Verification items for the finished model (mm, model axes). A direction names the side the tool comes from. Round coordinates to 2 decimals unless told otherwise and drop trailing zeros. Loops run counter-clockwise (first coordinate to the right, second up) from the corner with the lowest first, then second, coordinate; pieces in that order, holes last. Notation, with made-up numbers: (80.5, 50) -> (120.5, 50) arc R23 cw to (120.5, 63) -> close; hole circle Ø10 at (12, 26.25). An arc over 180 degrees is marked (long way). Write item = value, one per line. Start each with the question number.
```python
from build123d import *

# Parameters (mm, degrees)
BOSS_EXTRUDE1_DEPTH      = 20
BOSS_EXTRUDE2_DEPTH      = 12.7
BOSS_EXTRUDE2_DEPTH_BACK = 21.59
SKETCH2_R                = 5.710413334
CUT_EXTRUDE1_DEPTH       = 56.401981837


with BuildPart() as part:
    # Sketch1 → Boss-Extrude1 (new body)
    with BuildSketch(Plane(origin=(0, 0, 0), x_dir=(1, 0, 0), z_dir=(0, 1, 0))):
        Polygon((-32.500000024, -12.3), (-19.800000024, -25), (32.500000024, -25), (32.500000024, 25), (-32.500000024, 25), align=None)
    extrude(amount=BOSS_EXTRUDE1_DEPTH)

    # Sketch2 → Boss-Extrude2 (add, two sides: drawn at the far end of the back side and taken through both)
    with BuildSketch(Plane.ZY.offset(32.500000024).offset(-BOSS_EXTRUDE2_DEPTH_BACK)):
        with Locations((19.316364111, 10.795)):
            Circle(SKETCH2_R)
    extrude(amount=BOSS_EXTRUDE2_DEPTH + BOSS_EXTRUDE2_DEPTH_BACK)

    # Sketch3 → Cut-Extrude1 (cut, through all)
    with BuildSketch(Plane(origin=(0, 20, 0), x_dir=(1, 0, 0), z_dir=(0, 1, 0))):
        with BuildLine():
            Line((30.500000024, -19.5), (30.500000024, -21))
            ThreePointArc((30.500000024, -21), (28.500000024, -23), (26.500000024, -21))
            Line((26.500000024, -21), (26.500000024, -19.5))
            ThreePointArc((26.500000024, -19.5), (28.500000024, -17.5), (30.500000024, -19.5))
        make_face()
        with BuildLine():
            Line((-26.500000024, 21), (-26.500000024, 19.5))
            ThreePointArc((-26.500000024, 19.5), (-28.500000024, 17.5), (-30.500000024, 19.5))
            Line((-30.500000024, 19.5), (-30.500000024, 21))
            ThreePointArc((-30.500000024, 21), (-28.500000024, 23), (-26.500000024, 21))
        make_face()
    extrude(amount=-CUT_EXTRUDE1_DEPTH, mode=Mode.SUBTRACT)


solid = part.part
```
(1) Scan lines: line 1 (Z direction, x = 25, y = 7); line 2 (X direction, y = 19.25, z = 12); line 3 (Z direction, x = -40.5, y = 11.25). Record each from-to range of solid material in increasing order. Write a range as [from, to].
(2) Section check C-C on z = -8. Enter the section's corners in (x, y), then the cut area to 3 significant figures.
(3) Draft check along Y on faces 1 (the flat face through (0, 20, 0)), 2 (the cylindrical face through (-35.435, 12.51, 24.763)), 3 (the flat face through (-26.5, 10, -20)). Enter one of: +Y half, -Y half, draft (parallel to the pull), parting line (faces both ways), or undercut.
(4) Depth check by flat-ended pin: pin 1 Ø10 at (y, z) = (12.5, -9) entering from -X; pin 2 Ø3 at (x, y) = (-23.5, 4.5) entering from +Z; pin 3 Ø1.5 at (x, z) = (-28, 2.5) entering from -Y; pin 4 Ø1 at (x, y) = (16, 13.5) entering from +Z. Enter the tip coordinate at first touch or a pass-through.
(5) Access from +Z, -Z, +X, -X, +Y, -Y to the whole of each face (thin tool, end or side, straight path). Record for faces 4 (the flat face through (0, 10, -25)), 5 (the flat face through (-32.5, 10, -7)), 6 (the flat face through (30.5, 10, 20)).
(6) Section check B-B on y = 13. Enter the section's corners in (x, z).
(7) Section check A-A on x = 28.5. Enter the section's corners in (y, z), then the cut area to 3 significant figures.
(8) Section check D-D on x = -28. Enter the section's corners in (y, z) (1 decimal), then the cut area to 3 significant figures.
Computed values:
q1.line_1 = [-25, 25]
q1.line_2 = [-32.5, 32.5]
q1.line_3 = [13.62, 25.01]
q2.outline = (-32.5, 0) -> (32.5, 0) -> (32.5, 20) -> (-32.5, 20) -> close
q2.area = 1,300 mm²
q3.face_1 = +Y half
q3.face_2 = parting line
q3.face_3 = draft
q4.pin_1 = -32.5
q4.pin_2 = 22.8
q4.pin_3 = 0
q4.pin_4 = 25
q5.face_4 = -Z, +X, -X, +Y, -Y
q5.face_5 = -Z, -X, +Y, -Y
q5.face_6 = +Y, -Y
q6.outline = (-45.2, 14.05) -> (-30.75, 14.05) -> (-32.5, 12.3) -> (-32.5, -25) -> (32.5, -25) -> (32.5, 25) -> (-19.8, 25) -> (-20.22, 24.58) -> (-45.2, 24.58) -> close; hole (-30.5, -21) arc R2 ccw to (-26.5, -21) -> (-26.5, -19.5) arc R2 ccw to (-30.5, -19.5) -> close; hole (26.5, 19.5) arc R2 ccw to (30.5, 19.5) -> (30.5, 21) arc R2 ccw to (26.5, 21) -> close
q7.outline = (0, -25) -> (20, -25) -> (20, 17.5) -> (0, 17.5) -> close; (0, 23) -> (20, 23) -> (20, 25) -> (0, 25) -> close
q7.area = 890 mm²
q8.outline = (0, -25) -> (20, -25) -> (20, -22.9) -> (0, -22.9) -> close; (0, -17.6) -> (20, -17.6) -> (20, 16.8) -> (15.9, 16.8) arc R5.7 ccw (long way) to (5.7, 16.8) -> (0, 16.8) -> close
q8.area = 808 mm²
